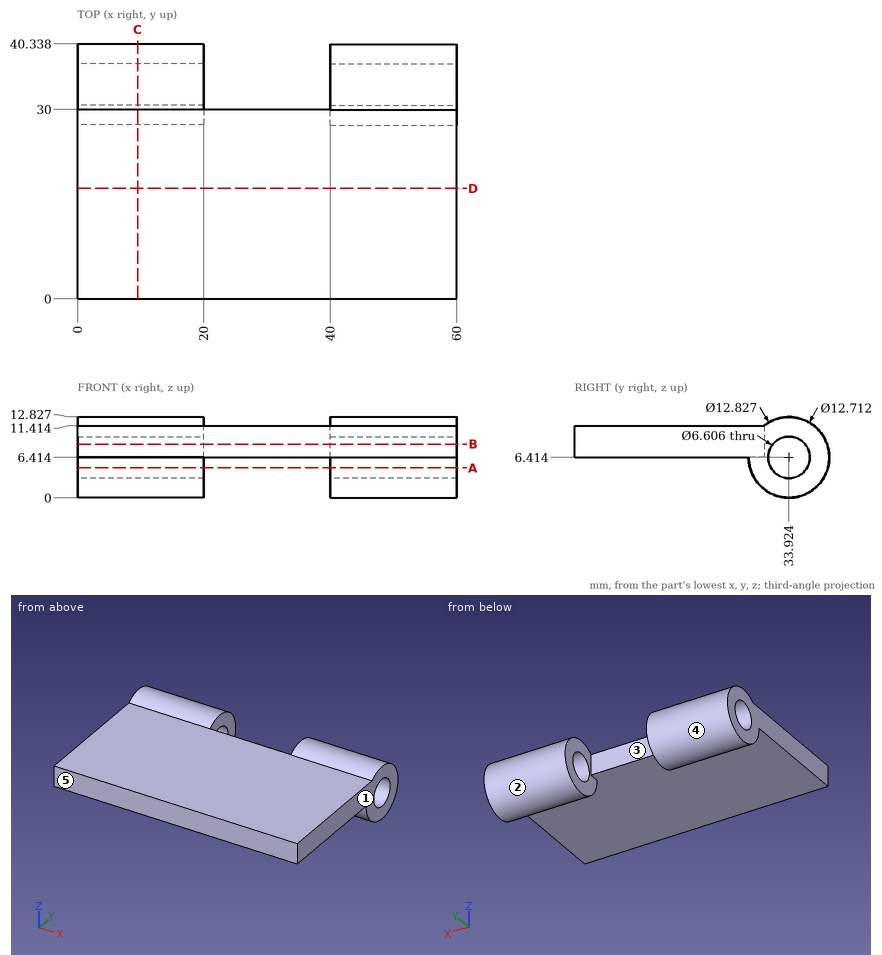
Job drawing, mm, ordinate dimensions from the low corner. One solid piece. A direction names the side the tool comes from. Coordinates: 2 decimals unless noted, no trailing zeros. Write each loop counter-clockwise with the first axis right and the second up, starting at its lowest first coordinate (ties: lowest second). Pieces come first, ordered by that corner, then holes. Notation, with made-up numbers: M 27.25,-30 L 32.25,-30 A22 ccw 32.25,-12 Z; hole C 15,-32.75 d3. An arc over 180 degrees is marked long. Answer as a JSON object with one key per item and string values. Group by question number.
1) Tool access for the marked faces 4 and 5: list every direction of +Z, -Z, +X, -X, +Y, -Y with a clear straight run to the whole face (end or side of a thin tool).
2) Saw through at D-D (y = 17.5). Write the cut outline in (x, z).
3) Saw through at A-A (z = 4.75). Write the cut outline in (x, y), plus the area to 3 significant figures.
4) Wall check: line 1 (Z direction, x = 23, y = 21.5); line 2 (Y direction, x = 28, z = 11.25); line 3 (Y direction, x = 46, z = 6.75). Give the ranges that are in metal, low to high. Write a range as from..to.
5) Pin check, flat tips, straight feed: pin 1 Ø2 at (x, y) = (16.5, 4.5) entering from -Z; pin 2 Ø1.5 at (x, z) = (41.5, 10) entering from +Y; pin 3 Ø4 at (x, z) = (25.5, 9) entering from +Y. Stop position of each tip, or through.
6) Saw through at C-C (x = 9.5). Write the cut outline in (y, z) (1 decimal).
7) Mould opens along X. For the marked faces 1, 2 and 3 say: +X half, -X half, draft (parallel to the pull), parting line (faces both ways), or undercut.
8) Saw through at B-B (z = 8.5). Write the cut outline in (x, y) (1 decimal), plus the area to 3 significant figures.
Values follow:
{
 "1": {"face 4": "-X", "face 5": "+Z, -Z, +X, -X, -Y"},
 "2": {"outline": "M 0,6.41 L 60,6.41 L 60,11.41 L 0,11.41 Z"},
 "3": {"outline": "M 0,27.79 L 20,27.79 L 20,31.07 L 0,31.07 Z; M 0,36.78 L 20,36.78 L 20,40.06 L 0,40.06 Z; M 40,27.73 L 60,27.73 L 60,31.07 L 40,31.07 Z; M 40,36.78 L 60,36.78 L 60,40.12 L 40,40.12 Z", "area": "265 mm2"},
 "4": {"line 1": "z = 6.41..11.41", "line 2": "y = 0..30", "line 3": "y = 0..30.64, 37.21..40.33"},
 "5": {"pin 1": "stops at z = 6.41", "pin 2": "stops at y = 39.68", "pin 3": "stops at y = 30"},
 "6": {"outline": "M 0,6.4 L 27.6,6.4 A6.4 ccw long 30,11.4 L 0,11.4 Z; hole C 33.9,6.4 d6.6"},
 "7": {"face 1": "+X half", "face 2": "draft", "face 3": "undercut"},
 "8": {"outline": "M 0,0 L 60,0 L 60,31.4 L 40,31.4 L 40,30 L 20,30 L 20,31.4 L 0,31.4 Z; M 0,36.5 L 20,36.5 L 20,39.9 L 0,39.9 Z; M 40,36.5 L 60,36.5 L 60,40 L 40,40 Z", "area": "1,990 mm2"}
}
